Work out the finished part from the listing and answer in its coordinate system (mm). Give positions to 0.01 mm unless a question says otherwise; leave off trailing zeros. Order: outer loops, then holes, each group sorted by start corner. A loop starts at its lowest first (then second) coordinate and runs counter-clockwise, first axis right, second up. Notation, with made-up numbers: (65.5, 32.25) - (74.5, 32.25) arc R12 cw to (74.5, 47.25) - close; hole circle Ø5 at (27, 3.5). An arc over 180 degrees is marked (long way). Write each question's results on one line, items separated by ' | '.
from build123d import *

# Parameters (mm, degrees)
REVOLVE1_ANGLE = 90


with BuildPart() as part:
    # Sketch1 → Revolve1 (revolve)
    with BuildSketch(Plane.XY):
        with BuildLine():
            Line((304.8, 0), (304.8, 914.4))
            ThreePointArc((304.8, 914.4), (215.526146906, 1129.926146906), (0, 1219.2))
            Line((0, 1219.2), (0, 1206.5))
            ThreePointArc((0, 1206.5), (206.545890785, 1120.945890785), (292.1, 914.4))
            Line((292.1, 914.4), (292.1, 0))
            ThreePointArc((292.1, 0), (206.545890785, -206.545890785), (0, -292.1))
            Line((0, -292.1), (0, -304.8))
            ThreePointArc((0, -304.8), (215.526146906, -215.526146906), (304.8, 0))
        make_face()
    revolve(axis=Axis((0, 1258.634144443, 0), (0, 1, 0)), revolution_arc=REVOLVE1_ANGLE)


solid = part.part
1. Determine the mould class of faces 1 (the face through (298, 517, 0)), 2 (the face through (208.804, 450.799, -204.262)) for opening direction Y: +Y half, -Y half, draft (parallel to the pull), parting line (faces both ways), or undercut.
Answer list:
face 1: draft | face 2: undercut
2. A cutting plane is placed at C-C, the plane y = 89. Write down the section's boundary in (x, z), then the cut area to 3 significant figures.
Answer list:
outline: (0, -304.8) arc R304.8 ccw to (304.8, 0) - (292.1, 0) arc R292.1 cw to (0, -292.1) - close | area: 5,950 mm^2
3. Given P1, Ø2, axis at y = 726, z = -192, coming from the +X side; P2, Ø12, axis at x = 208, z = -39.5, coming from the -Y side; P3, Ø10, axis at x = 55.5, y = 666, coming from the +Z side, each flat-ended and moving along its own axis, determine where each tip first touches the part or whether it passes through.
Answer list:
P1: x = 237.53 | P2: y = -224.91 | P3: z = -285.77
4. Straight lines are drawn through the part: line 1 (Y direction, x = 137.5, z = -217.5); line 2 (Y direction, x = 18, z = -92); line 3 (X direction, y = 66.5, z = -261). For each, find the intervals that lie inside material, in ascending order. Write a range as [from, to].
Answer list:
line 1: [-163.37, -138.24], [1052.64, 1077.77] | line 2: [-290.03, -276.65], [1191.05, 1204.43] | line 3: [131.15, 157.42]
5. A cutting plane is placed at A-A, the plane x = 144. Write down the section's boundary in (y, z).
Answer list:
outline: (-268.64, 0) arc R268.64 ccw to (0, -268.64) - (914.4, -268.64) arc R268.64 ccw to (1183.04, 0) - (1168.54, 0) arc R254.14 cw to (914.4, -254.14) - (0, -254.14) arc R254.14 cw to (-254.14, 0) - close
6. A cutting plane is placed at B-B, the plane z = -141. Write down the section's boundary in (x, y), then the cut area to 3 significant figures.
Answer list:
outline: (0, -270.23) arc R270.23 ccw to (270.23, 0) - (270.23, 914.4) arc R270.23 ccw to (0, 1184.63) - (0, 1170.22) arc R255.82 cw to (255.82, 914.4) - (255.82, 0) arc R255.82 cw to (0, -255.82) - close | area: 25,100 mm^2
